Autodesk Inventor part; units mm, degrees
ref_plane "YZ Plane" through (0, 0, 0) normal (1, 0, 0) x (0, 1, 0)
ref_plane "XZ Plane" through (0, 0, 0) normal (0, 1, 0) x (-1, 0, 0)
ref_plane "XY Plane" through (0, 0, 0) normal (0, 0, 1) x (1, 0, 0)
sketch "Esquisse1" plane through (0, 0, 0) normal (0, 0, 1) x (1, 0, 0)
  line L0 (10, 0) -> (104.4, 0)
  line L1 (114.4, -10) -> (114.4, -105.15)
  line L2 (104.4, -115.15) -> (49, -115.15)
  line L3 (0, -115.15) -> (0, -10)
  line L4 (0, -115.15) -> (0, -160.65)
  line L5 (39, -160.65) -> (39, -125.15)
  arc A0 (0, -160.65) -> (39, -160.65) centre (19.5, -160.65) ccw
  line L6 (0, -10) -> (0, 0)
  line L7 (10, 0) -> (0, 0)
  line L8 (114.4, -10) -> (114.4, 0)
  line L9 (114.4, 0) -> (104.4, 0)
  line L10 (114.4, -105.15) -> (114.4, -115.15)
  line L11 (104.4, -115.15) -> (114.4, -115.15)
  line L12 (39, -125.15) -> (39, -115.15)
  line L13 (49, -115.15) -> (39, -115.15)
  dimension "d0" = 39
  dimension "d1" = 114.4
  dimension "d2" = 45.5
  dimension "d3" = 115.15
extrude "Extrusion1" add sketch "Esquisse1" along normal blind 5
sketch "Esquisse2" plane through (0, 0, 5) normal (0, 0, 1) x (1, 0, 0)
  line L0 (31.7, -46.85) -> (31.7, -87.85)
  line L1 (11.7, -87.85) -> (11.7, -46.85)
  line L2 (102.7, -26.7) -> (102.7, -67.7)
  line L3 (82.7, -67.7) -> (82.7, -26.7)
  line L4 (0, 0) -> (0, -160.65)
  line L5 (114.4, -115.15) -> (114.4, 0)
  circle A0 centre (16.7, -42.46) radius 2.5
  circle A1 centre (26.7, -42.46) radius 2.5
  circle A2 centre (16.7, -92.24) radius 2.5
  circle A3 centre (26.7, -92.24) radius 2.5
  circle A4 centre (87.7, -72.09) radius 2.5
  circle A5 centre (97.7, -72.09) radius 2.5
  circle A6 centre (87.7, -22.31) radius 2.5
  circle A7 centre (97.7, -22.31) radius 2.5
  circle A8 centre (19.5, -160.65) radius 5
  line L6 (114.4, 0) -> (0, 0)
  line L7 (39, -115.15) -> (114.4, -115.15)
  line L8 (22.7, -46.85) -> (22.7, -39.35)
  line L9 (22.7, -39.35) -> (20.7, -39.35)
  line L10 (20.7, -39.35) -> (20.7, -46.85)
  line L11 (93.7, -67.7) -> (93.7, -75.2)
  line L12 (91.7, -75.2) -> (91.7, -67.7)
  line L13 (93.7, -26.7) -> (93.7, -19.2)
  line L14 (93.7, -19.2) -> (91.7, -19.2)
  line L15 (91.7, -19.2) -> (91.7, -26.7)
  line L16 (11.7, -46.85) -> (20.7, -46.85)
  line L17 (31.7, -46.85) -> (22.7, -46.85)
  line L18 (22.7, -87.85) -> (22.7, -95.35)
  line L19 (22.7, -95.35) -> (20.7, -95.35)
  line L20 (20.7, -95.35) -> (20.7, -87.85)
  line L21 (11.7, -87.85) -> (20.7, -87.85)
  line L22 (22.7, -87.85) -> (31.7, -87.85)
  line L23 (82.7, -26.7) -> (91.7, -26.7)
  line L24 (93.7, -26.7) -> (102.7, -26.7)
  line L25 (82.7, -67.7) -> (91.7, -67.7)
  line L26 (93.7, -67.7) -> (102.7, -67.7)
  line L27 (91.7, -75.2) -> (93.7, -75.2)
  point P0 (0, -10)
  point P1 (114.4, -105.15)
  point P2 (114.4, -10)
  point P3 (39, -160.65)
  point P4 (104.4, 0)
  point P5 (10, 0)
  point P6 (49, -115.15)
  point P7 (104.4, -115.15)
  dimension "d7" = 11.7
  dimension "d8" = 11.7
  dimension "d9" = 20
  dimension "d10" = 20
  dimension "d11" = 41
  dimension "d12" = 41
  dimension "d13" = 10
  dimension "d14" = 19.5
  dimension "d16" = 5
  dimension "d18" = 5
  dimension "d20" = 10
  dimension "d21" = 5
  dimension "d22" = 5
  dimension "d26" = 10
  dimension "d28" = 5
  dimension "d31" = 5
  dimension "d32" = 10
  dimension "d33" = 5
  dimension "d36" = 5
  dimension "d37" = 10
  dimension "d41" = 9
  dimension "d43" = 4.39
  dimension "d44" = 4.39
  dimension "d45" = 5
  dimension "d46" = 7.5
  dimension "d47" = 7.5
  dimension "d48" = 9
  dimension "d49" = 9
  dimension "d50" = 9
  dimension "d51" = 5
  dimension "d52" = 4.39
  dimension "d53" = 4.39
  dimension "d54" = 7.5
  dimension "d55" = 9
  dimension "d56" = 9
  dimension "d57" = 4.39
  dimension "d58" = 4.39
  dimension "d59" = 5
  dimension "d60" = 9
  dimension "d61" = 9
  dimension "d62" = 7.5
  dimension "d63" = 4.39
  dimension "d64" = 4.39
  dimension "d65" = 5
  dimension "d168" = 41
  dimension "d169" = 41
extrude "Extrusion2" cut sketch "Esquisse2" against normal blind 5
sketch "Esquisse3" plane through (39, -115.15, 0) normal (0, -1, 0) x (1, 0, 0)
  line L0 (0, 0) -> (75.4, 0)
  line L1 (0, 0) -> (75.4, 0)
  line L2 (75.4, 0) -> (75.4, -54.86)
  line L3 (75.4, -54.86) -> (0, -54.86)
  line L4 (0, -54.86) -> (0, 0)
  point P0 (-39, 0)
  dimension "d68" = 54.86
extrude "Extrusion3" add sketch "Esquisse3" against normal blind 5
sketch "Esquisse4" plane through (0, 0, 5) normal (0, 0, 1) x (1, 0, 0)
  line L0 (44.7, -55.15) -> (49.7, -40.15)
  line L1 (49.7, -40.15) -> (49.7, -90.15)
  line L2 (49.7, -90.15) -> (44.7, -105.15)
  line L3 (44.7, -105.15) -> (44.7, -55.15)
  line L4 (0, 0) -> (0, -160.65)
  line L5 (54.7, -40) -> (59.7, -25)
  line L6 (59.7, -25) -> (59.7, -75)
  line L7 (59.7, -75) -> (54.7, -90)
  line L8 (54.7, -90) -> (54.7, -40)
  line L9 (64.7, -25) -> (69.7, -10)
  line L10 (69.7, -10) -> (69.7, -60)
  line L11 (69.7, -60) -> (64.7, -75)
  line L12 (64.7, -75) -> (64.7, -25)
  line L13 (114.4, 0) -> (0, 0)
  line L14 (39, -115.15) -> (114.4, -115.15)
  dimension "d71" = 50
  dimension "d72" = 50
  dimension "d73" = 15
  dimension "d74" = 15
  dimension "d75" = 5
  dimension "d78" = 44.7
  dimension "d79" = 50
  dimension "d80" = 50
  dimension "d81" = 15
  dimension "d82" = 15
  dimension "d83" = 5
  dimension "d84" = 54.7
  dimension "d85" = 50
  dimension "d86" = 50
  dimension "d87" = 15
  dimension "d88" = 15
  dimension "d89" = 5
  dimension "d90" = 64.7
  dimension "d91" = 10
  dimension "d92" = 10
  dimension "d93" = 25
extrude "Extrusion4" cut sketch "Esquisse4" against normal blind 5
sketch "Esquisse5" plane through (39, -115.15, 5) normal (0, -1, 0) x (1, 0, 0)
  line L0 (17.2, -20) -> (58.2, -20)
  line L1 (58.2, -40) -> (17.2, -40)
  circle A0 centre (12.81, -25) radius 2.5
  circle A1 centre (12.81, -35) radius 2.5
  circle A2 centre (62.59, -25) radius 2.5
  circle A3 centre (62.59, -35) radius 2.5
  line L2 (0, 0) -> (75.4, 0)
  line L3 (0, -59.86) -> (0, -5)
  line L4 (17.2, -31) -> (9.7, -31)
  line L5 (9.7, -31) -> (9.7, -29)
  line L6 (9.7, -29) -> (17.2, -29)
  line L7 (58.2, -29) -> (65.7, -29)
  line L8 (65.7, -29) -> (65.7, -31)
  line L9 (65.7, -31) -> (58.2, -31)
  line L10 (17.2, -29) -> (17.2, -20)
  line L11 (17.2, -31) -> (17.2, -40)
  line L12 (58.2, -40) -> (58.2, -31)
  line L13 (58.2, -29) -> (58.2, -20)
  line L14 (75.4, -59.86) -> (75.4, 0)
  point P0 (-39, -5)
  dimension "d96" = 5
  dimension "d98" = 5
  dimension "d99" = 5
  dimension "d100" = 20
  dimension "d101" = 41
  dimension "d103" = 20
  dimension "d109" = 10
  dimension "d110" = 10
  dimension "d111" = 5
  dimension "d112" = 5
  dimension "d113" = 5
  dimension "d114" = 9
  dimension "d115" = 9
  dimension "d116" = 9
  dimension "d117" = 9
  dimension "d118" = 7.5
  dimension "d119" = 7.5
  dimension "d170" = 41
  dimension "d171" = 17.2
  dimension "d172" = 4.39
  dimension "d173" = 4.39
  dimension "d174" = 4.39
  dimension "d175" = 4.39
  dimension "d176" = 17.2
extrude "Extrusion5" cut sketch "Esquisse5" against normal blind 5
chamfer "Chanfrein1" distance 5 angle 45 1 edges at (39, -115.15, 2.5)
sketch "Esquisse7" plane through (114.4, -115.15, -54.86) normal (0, 0, -1) x (-1, 0, 0)
  line L0 (0, 0) -> (75.4, 0)
  line L1 (75.4, 0) -> (36.4, 0)
  line L2 (36.4, 0) -> (36.4, -65)
  line L3 (36.4, -65) -> (75.4, -65)
  line L4 (75.4, -65) -> (94.9, -65)
  arc A0 (94.9, -65) -> (94.9, -26) centre (94.9, -45.5) ccw
  line L5 (94.9, -26) -> (75.4, -26)
  line L6 (75.4, 0) -> (75.4, -26)
  point P0 (114.4, 115.15)
  dimension "d129" = 39
  dimension "d130" = 65
  dimension "d131" = 19.5
extrude "Extrusion6" add sketch "Esquisse7" against normal blind 5
sketch "Esquisse8" plane through (114.4, -110.15, -54.86) normal (0, 0, -1) x (-1, 0, 0)
  circle A0 centre (94.9, -50.5) radius 5
  circle A1 centre (94.9, -50.5) radius 5
  point P0 (114.4, 110.15)
extrude "Extrusion7" cut sketch "Esquisse8" against normal blind 5
sketch "Esquisse9" plane through (0, 0, 0) normal (0, 1, 0) x (1, 0, 0)
  line L0 (0, 0) -> (75.4, 0)
  line L1 (75.4, 0) -> (75.4, 42.9)
  line L2 (75.4, 42.9) -> (0, 42.9)
  line L3 (0, 42.9) -> (0, 0)
  point P0 (114.4, 0)
  dimension "d137" = 39
  dimension "d138" = 42.9
extrude "Extrusion8" add sketch "Esquisse9" against normal blind 5
sketch "Esquisse10" plane through (0, 0, 5) normal (0, 1, 0) x (1, 0, 0)
  line L0 (58.2, 39.9) -> (17.2, 39.9)
  line L1 (17.2, 19.9) -> (58.2, 19.9)
  circle A0 centre (62.59, 34.9) radius 2.5
  circle A1 centre (62.59, 24.9) radius 2.5
  circle A2 centre (12.81, 34.9) radius 2.5
  circle A3 centre (12.81, 24.9) radius 2.5
  line L2 (75.4, 5) -> (75.4, 47.9)
  line L3 (58.2, 30.9) -> (65.7, 30.9)
  line L4 (65.7, 30.9) -> (65.7, 28.9)
  line L5 (65.7, 28.9) -> (58.2, 28.9)
  line L6 (17.2, 30.9) -> (9.7, 30.9)
  line L7 (9.7, 30.9) -> (9.7, 28.9)
  line L8 (9.7, 28.9) -> (17.2, 28.9)
  line L9 (58.2, 39.9) -> (58.2, 30.9)
  line L10 (58.2, 28.9) -> (58.2, 19.9)
  line L11 (17.2, 39.9) -> (17.2, 30.9)
  line L12 (17.2, 28.9) -> (17.2, 19.9)
  line L13 (0, 47.9) -> (0, 0)
  line L14 (75.4, 47.9) -> (0, 47.9)
  point P0 (0, 5)
  dimension "d141" = 41
  dimension "d142" = 20
  dimension "d143" = 5
  dimension "d144" = 5
  dimension "d145" = 5
  dimension "d146" = 5
  dimension "d151" = 10
  dimension "d152" = 5
  dimension "d154" = 10
  dimension "d156" = 5
  dimension "d157" = 9
  dimension "d158" = 9
  dimension "d159" = 7.5
  dimension "d160" = 7.5
  dimension "d161" = 17.2
  dimension "d162" = 17.2
  dimension "d163" = 4.39
  dimension "d164" = 17.2
  dimension "d167" = 8
  dimension "d177" = 4.39
  dimension "d178" = 4.39
  dimension "d179" = 4.39
extrude "Extrusion9" cut sketch "Esquisse10" against normal blind 5
fillet "Congé1" radius 5 1 edges at (37.7, -5, 0)
fillet "Congé2" radius 5 1 edges at (76.7, -110.15, 0)
fillet "Congé3" radius 5 1 edges at (58.5, -115.15, -49.86)
properties part number "Rbiceps" material "Plastique ABS"
Source: CAD feature listing. Evaluate the final solid. Frame: model axes, mm. A direction names the side the tool comes from. Give positions to 0.01 mm unless a question says otherwise; leave off trailing zeros. Write each loop counter-clockwise with the first axis right and the second up, starting at its lowest first coordinate (ties: lowest second). Pieces come first, ordered by that corner, then holes. Notation, with made-up numbers: (-15, 36) -> (-10, 36) arc R27 ccw to (-10, 57) -> close; hole circle Ø4 at (44.25, 27.5). An arc over 180 degrees is marked (long way). Return JSON: item names as keys, results as strings. Group by question number.
1. Mould query, pull axis X, two halves, no side actions, for faces 6 (the face through (14, -2, -25.9)), 7 (the face through (77.23, -108.65, -1.43)), 8 (the face through (114.4, -75, 2)). Classes: +X half, -X half, draft (parallel to the pull), parting line (faces both ways), or undercut.
2. Material intervals for line 1 (Z direction, x = 51.81, y = -111.3); line 2 (X direction, y = -3.25, z = -29.9); line 3 (Z direction, x = 101, y = -111), sorted ascending. Write a range as from..to.
3. Pin query (flat end, axial travel): pin 1 Ø12 at (x, z) = (49.5, -42) entering from -Y; pin 2 Ø12 at (x, y) = (44, -24.5) entering from -Z; pin 3 Ø1 at (x, z) = (97, -40) entering from +Y. Return the tip coordinate at first contact, or that it passes through.
4. Access query for faces 1 (the face through (19.929, -180.145, 2.465)), 2 (the face through (29, -141.15, -52)), 3 (the face through (101, -113, -24)), 4 (the face through (20.7, -92, 3)), 5 (the face through (77, -113, -35)). Directions: +Z, -Z, +X, -X, +Y, -Y. A direction counts if a zero-diameter tool reaches every point of the face in a straight line with its end or side. Return the directions, or none.
5. Section B-B, the plane y = -42.46. Count the separate pieces of the cut face and the enclosed holes in it, then the cut area to 3 significant figures.
6. Section A-A, the plane y = -131.5. Output: boundary loops of the cut face in (x, z), then the cut area to 3 significant figures.
7. Section D-D, the plane y = -92.24. Output: boundary loops of the cut face in (x, z), then the cut area to 3 significant figures.
8. Section C-C, the plane y = -112.5. Output: boundary loops of the cut face in (x, z), then the cut area to 3 significant figures.
Determined:
{
 "1": {"face 6": "undercut", "face 7": "draft", "face 8": "+X half"},
 "2": {"line 1": "z = -54.86..-32.5, -27.5..-26, -24..-22.5, -17.5..5", "line 2": "x = 0..10.31, 15.31..17.2, 58.2..60.09, 65.09..75.4", "line 3": "z = -54.86..-32.43, -27.57..-26, -24..-22.43, -17.57..5"},
 "3": {"pin 1": "stops at y = -116.26", "pin 2": "stops at z = 0", "pin 3": "stops at y = -110.15"},
 "4": {"face 1": "+Z, -Y", "face 2": "-Z, -X, +Y", "face 3": "+Y, -Y", "face 4": "+Z, -Z", "face 5": "-Y"},
 "5": {"separate pieces": "8", "enclosed holes": "0", "area": "358 mm2"},
 "6": {"outline": "(0, 0) -> (39, 0) -> (39, 5) -> (0, 5) -> close; (39, -54.86) -> (78, -54.86) -> (78, -49.86) -> (39, -49.86) -> close", "area": "390 mm2"},
 "7": {"outline": "(0, 0) -> (14.2, 0) -> (14.2, 5) -> (0, 5) -> close; (19.2, 0) -> (20.7, 0) -> (20.7, 5) -> (19.2, 5) -> close; (22.7, 0) -> (24.2, 0) -> (24.2, 5) -> (22.7, 5) -> close; (29.2, 0) -> (44.7, 0) -> (44.7, 5) -> (29.2, 5) -> close; (49, 0) -> (114.4, 0) -> (114.4, 5) -> (49, 5) -> close", "area": "490 mm2"},
 "8": {"outline": "(0, 0) -> (39, 0) -> (39, -54.86) -> (114.4, -54.86) -> (114.4, 5) -> (0, 5) -> close; hole (48.7, -26) -> (56.2, -26) -> (56.2, -35) -> (97.2, -35) -> (97.2, -26) -> (104.7, -26) -> (104.7, -24) -> (97.2, -24) -> (97.2, -15) -> (56.2, -15) -> (56.2, -24) -> (48.7, -24) -> close; hole circle Ø5 at (51.81, -30); hole circle Ø5 at (51.81, -20); hole circle Ø5 at (101.59, -30); hole circle Ø5 at (101.59, -20)", "area": "3,780 mm2"}
}
